```python
from build123d import *

# Parameters (mm, degrees)
F1_DEPTH = 50.8
F3_DEPTH = 12.7
F5_DEPTH = 12.7
F7_DEPTH = 76.201
F8_R     = 12.7


with BuildPart() as f1:
    # F0 (on Front) → F1 (new body)
    with BuildSketch(Plane.XZ):
        Polygon((0, 38.1), (0, 0), (76.2, 0), (76.2, 12.7), (48.502727, 12.7), (48.502727, 38.1), (35.802727, 38.1), (35.802727, 50.8), (10.402727, 50.8), align=None)
    extrude(amount=F1_DEPTH)

    # F2 (on face) → F3 (cut)
    with BuildSketch(Plane.XZ.offset(50.8)):
        Polygon((35.802727, 50.8), (23.102727, 50.8), (23.102727, 25.400003), (48.502727, 25.4), (48.502727, 38.1), (35.802727, 38.1), align=None)
    extrude(amount=-F3_DEPTH, mode=Mode.SUBTRACT)

    # F4 (on face) → F5 (cut)
    with BuildSketch(Plane(origin=(0, 0, 0), x_dir=(-1, 0, 0), z_dir=(0, 1, 0))):
        Polygon((-23.102727, 25.4), (-23.102727, 50.8), (-35.802727, 50.8), (-35.802727, 38.1), (-48.502727, 38.1), (-48.502727, 25.4), align=None)
    extrude(amount=-F5_DEPTH, mode=Mode.SUBTRACT)

    # F6 (on face) → F7 (cut, through all)
    with BuildSketch(Plane.YZ.offset(76.2)):
        with BuildLine():
            ThreePointArc((-31.75, 12.7), (-25.4, 6.35), (-19.05, 12.7))
            Line((-19.05, 12.7), (-31.75, 12.7))
        make_face()
        with BuildLine():
            Line((-31.75, 12.7), (-19.05, 12.7))
            ThreePointArc((-19.05, 12.7), (-25.4, 19.05), (-31.75, 12.7))
        make_face()
    extrude(amount=-F7_DEPTH, mode=Mode.SUBTRACT)

    # F8
    f8_edges = [f1.edges().sort_by_distance(p)[0] for p in [
        (76.2, -50.8, 6.35),
        (76.2, 0, 6.35),
    ]]
    fillet(f8_edges, radius=F8_R)


solid = f1.part
```
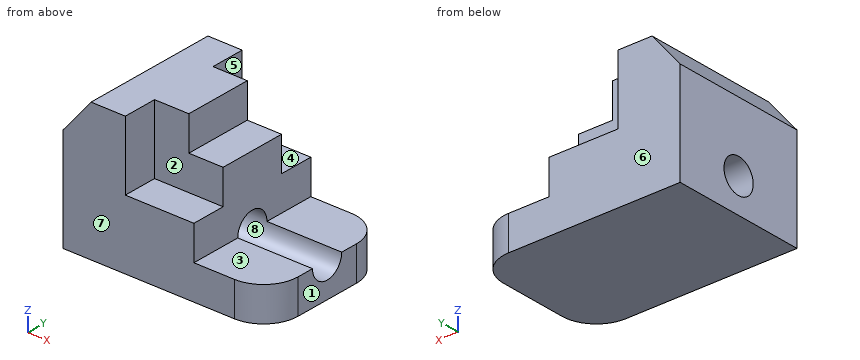
The model under review builds one solid part; all positions refer to its coordinate system, in mm. Face numbers are marked on the shaded views. A direction names the side the tool comes from. Round coordinates to 2 decimals unless told otherwise and drop trailing zeros. Write each loop counter-clockwise with the first axis right and the second up, starting at its lowest first coordinate (ties: lowest second). Pieces come first, ordered by that corner, then holes. Notation, with made-up numbers: (3.25, 2) -> (34.25, 2) arc R19 cw to (34.25, 18) -> close; hole circle Ø1 at (35, 3.5). An arc over 180 degrees is marked (long way). Use CSV: the item, a comma, the result in double quotes.
Q1. Consider section A-A (x = 30). Give the boundary of the cut face in (y, z).
Checks:
outline,"(-50.8, 0) -> (0, 0) -> (0, 25.4) -> (-12.7, 25.4) -> (-12.7, 50.8) -> (-38.1, 50.8) -> (-38.1, 25.4) -> (-50.8, 25.4) -> close; hole circle Ø12.7 at (-25.4, 12.7)"
Q2. Consider section C-C (z = 37). Give the boundary of the cut face in (x, y).
Checks:
outline,"(0, -50.8) -> (23.1, -50.8) -> (23.1, -38.1) -> (48.5, -38.1) -> (48.5, -12.7) -> (23.1, -12.7) -> (23.1, 0) -> (0, 0) -> close"
Q3. Mouldability with a two-part tool opening along Y and no side actions: class the marked faces 5, 6, 7 and 8 as released by +Y, released by -Y, zero draft, split by the parting line, or undercut.
Checks:
face 5,"zero draft"
face 6,"released by +Y"
face 7,"released by -Y"
face 8,"undercut"
Q4. For the marked faces 1, 2, 3 and 4, list the 3-axis set-ups (+Z, -Z, +X, -X, +Y, -Y) from which the entire face can be reached by the end or side of a thin tool; tool diameter is ignored.
Checks:
face 1,"+Z, -Z, +X, +Y, -Y"
face 2,"+Z, +X, -Y"
face 3,"+Z, +X, +Y, -Y"
face 4,"+Z, +X, +Y"
Q5. To check wall thickness, follow probe 1 along Z at (x, y) = (24, -25.4); probe 2 along Y at (x, z) = (36, 12.7); probe 3 along Z at (x, y) = (36, -25.4). State the ranges of each line that lie inside material, in increasing order. Write a range as [from, to].
Checks:
probe 1,"[0, 6.35], [19.05, 50.8]"
probe 2,"[-50.8, -31.75], [-19.05, 0]"
probe 3,"[0, 6.35], [19.05, 38.1]"
Q6. Consider section D-D (x = 19). Give the boundary of the cut face in (y, z), then the cut area to 3 significant figures.
Checks:
outline,"(-50.8, 0) -> (0, 0) -> (0, 50.8) -> (-50.8, 50.8) -> close; hole circle Ø12.7 at (-25.4, 12.7)"
area,"2,450 mm²"
Q7. Consider section B-B (y = -25.4). Give the boundary of the cut face in (x, z), then the cut area to 3 significant figures.
Checks:
outline,"(0, 0) -> (76.2, 0) -> (76.2, 6.35) -> (0, 6.35) -> close; (0, 19.05) -> (48.5, 19.05) -> (48.5, 38.1) -> (35.8, 38.1) -> (35.8, 50.8) -> (10.4, 50.8) -> (0, 38.1) -> close"
area,"1,800 mm²"
Q8. For pin 1 Ø4 at (y, z) = (-45, 32.5) entering from +X; pin 2 Ø20.5 at (x, z) = (33, 32.5) entering from -Y; pin 3 Ø2 at (y, z) = (-27, 39.5) entering from -X; pin 4 Ø6.5 at (x, y) = (40.5, -44.5) entering from +Z, all flat-tipped, find the tip position at first contact; note any pin that passes through.
Checks:
pin 1,"x = 23.1"
pin 2,"y = -50.8"
pin 3,"x = 0.33"
pin 4,"z = 25.4"
